from build123d import *

# Parameters (mm, degrees)
SKETCH4_W           = 35
SKETCH4_H           = 35
BOSS_EXTRUDE2_DEPTH = 35
SKETCH5_OUTSIDE_W   = 49.124
SKETCH5_OUTSIDE_H   = 49.124
SKETCH5_OUTSIDE_W_2 = 35
SKETCH5_OUTSIDE_H_2 = 35
SKETCH5_OUTSIDE_W_3 = 30
SKETCH5_OUTSIDE_H_3 = 30
CUT_EXTRUDE2_DEPTH  = 32.5


with BuildPart() as part:
    # Sketch4 → Boss-Extrude2 (new body)
    with BuildSketch(Plane.XY):
        with Locations((-2.784904398, 3.060708191)):
            Rectangle(SKETCH4_W, SKETCH4_H)
    extrude(amount=BOSS_EXTRUDE2_DEPTH)

    # Sketch5 outside → Cut-Extrude2 (cut)
    # profile 1 of 2: a face of its own
    with BuildSketch(Plane.XY.offset(35)):
        with Locations((-2.785, 3.061)):
            Rectangle(SKETCH5_OUTSIDE_W, SKETCH5_OUTSIDE_H)
        with Locations((-2.784904398, 3.060708191)):
            Rectangle(SKETCH5_OUTSIDE_W_2, SKETCH5_OUTSIDE_H_2, mode=Mode.SUBTRACT)
    # profile 2 of 2: a face of its own
    with BuildSketch(Plane.XY.offset(35)):
        with Locations((-2.784904398, 3.060708191)):
            Rectangle(SKETCH5_OUTSIDE_W_3, SKETCH5_OUTSIDE_H_3)
    extrude(amount=-CUT_EXTRUDE2_DEPTH, mode=Mode.SUBTRACT)


solid = part.part
Source: CAD feature listing. Evaluate the final solid. Frame: model axes, mm. A direction names the side the tool comes from. Round coordinates to 2 decimals unless told otherwise and drop trailing zeros. Write each loop counter-clockwise with the first axis right and the second up, starting at its lowest first coordinate (ties: lowest second). Pieces come first, ordered by that corner, then holes. Notation, with made-up numbers: M 12,-32.5 L 58,-32.5 A17 ccw 58,-15.5 Z; hole C 48,58.5 d3. An arc over 180 degrees is marked long. One line per item, written item: value. Start each with the question number.
Item 1: Section query A-A (z = 25). Return the cut outline in (x, y), plus the area to 3 significant figures.
Item 2: Mould query, pull axis Y, two halves, no side actions, for faces 1 (the flat face through (-3, 3, 0)), 2 (the flat face through (-3, 18.061, 19)), 3 (the flat face through (-3, 20.561, 17)). Classes: pulls with the +Y half, pulls with the -Y half, needs draft (parallel to the pull), parting line crosses it, or undercut.
Item 3: Ray query, L1, parallel to X at y = 7, z = 16.5; L2, parallel to Y at x = -5.5, z = 28; L3, parallel to Z at x = 3.5, y = 7.5. Return the intervals inside material, ascending. Write a range as from..to.
Item 4: Pin query (flat end, axial travel): pin 1 (1 mm diameter, centred on x = -10, y = 15.5, fed in from +Z). Return the tip coordinate at first contact, or that it passes through.
Item 5: Section query B-B (y = -0.5). Return the cut outline in (x, z).
Item 6: Set-up query: faces 4 (the flat face through (-3, -11.939, 19)), 5 (the flat face through (14.715, 3, 17)). Return all of +Z, -Z, +X, -X, +Y, -Y with unobstructed straight access to the full face (end or side cutting, diameter ignored); none if empty.
Item 7: Section query C-C (x = -10). Return the cut outline in (y, z).
Result set:
1. outline: M -20.28,-14.44 L 14.72,-14.44 L 14.72,20.56 L -20.28,20.56 Z; hole M -17.78,-11.94 L 12.22,-11.94 L 12.22,18.06 L -17.78,18.06 Z
1. area: 325 mm²
2. face 1: needs draft
2. face 2: undercut
2. face 3: pulls with the +Y half
3. L1: x = -20.28..-17.78, 12.22..14.72
3. L2: y = -14.44..-11.94, 18.06..20.56
3. L3: z = 0..2.5
4. pin 1: stops at z = 2.5
5. outline: M -20.28,0 L 14.72,0 L 14.72,35 L 12.22,35 L 12.22,2.5 L -17.78,2.5 L -17.78,35 L -20.28,35 Z
6. face 4: +Z
6. face 5: +Z, -Z, +X, +Y, -Y
7. outline: M -14.44,0 L 20.56,0 L 20.56,35 L 18.06,35 L 18.06,2.5 L -11.94,2.5 L -11.94,35 L -14.44,35 Z
